Could you check a few things on this drawing? It's one solid part, dimensions in mm from its lowest x, y, z. A direction names the side the tool comes from. Round coordinates to 2 decimals unless told otherwise and drop trailing zeros. Write each loop counter-clockwise with the first axis right and the second up, starting at its lowest first coordinate (ties: lowest second). Pieces come first, ordered by that corner, then holes. Notation, with made-up numbers: (56, 8) -> (70, 8) arc R21 ccw to (70, 36) -> close; hole circle Ø9 at (39.25, -22.5). An arc over 180 degrees is marked (long way). Answer in a Markdown table with one row per item. Add a question column.
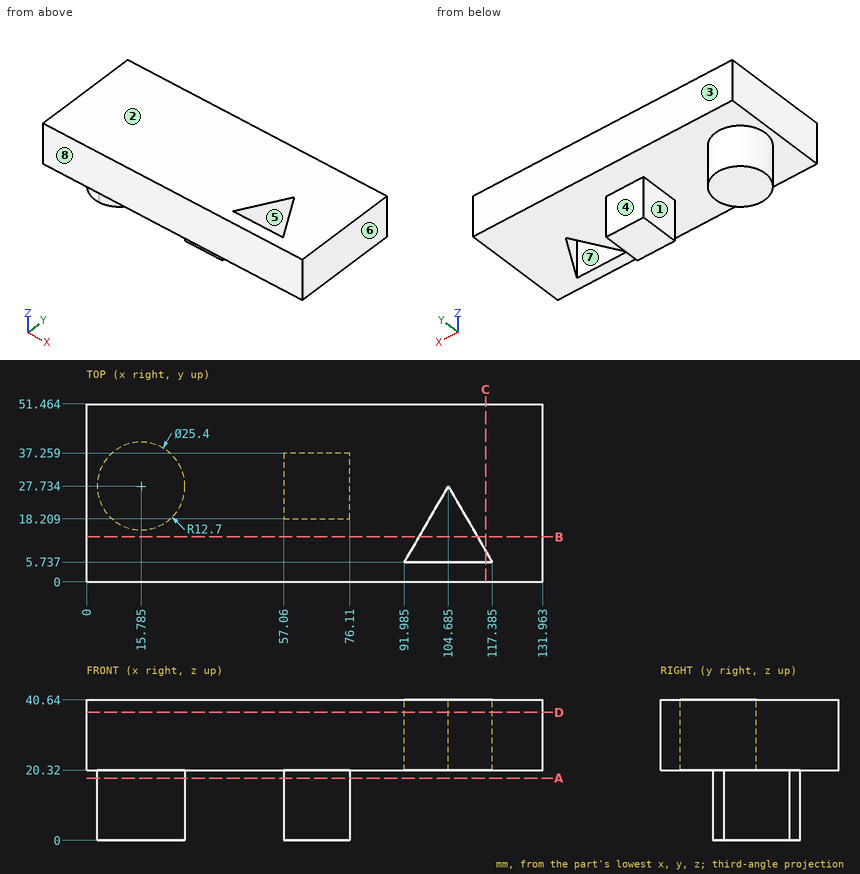
(1) I need wall thicknesses on L1, parallel to Z at x = 80.5, y = 32.5; L2, parallel to X at y = 24.5, z = 26.5; L3, parallel to X at y = 21, z = 3. Which ranges of each line are inside material? Lowest first, please.
(2) Suppose I cut it at D-D, the plane z = 37. Please give me the cut outline in (x, y) (1 decimal).
(3) For P1, Ø5, axis at y = 26.5, z = 17, coming from the -X side (1 decimal); P2, Ø15, axis at y = 25.5, z = 8, coming from the +X side; P3, Ø5.5, axis at x = 66.5, z = 7.5, coming from the -Y side, each with a flat end and sliding along its axis, tell me the tip position at first contact or that it passes through.
(4) If we mould it in two halves opening along Y, with no side actions, what happens to the marked faces 6, 7 and 8? For each: pulls with the +Y half, pulls with the -Y half, needs draft (parallel to the pull), parting line crosses it, or undercut.
(5) On a 3-axis mill with a long thin cutter (end or side, diameter ignored), from which of +Z, -Z, +X, -X, +Y, -Y can I reach the whole of each face in a straight line? I mean the marked faces 1, 2, 3, 4 and 5. Say none if no direction works.
(6) Suppose I cut it at B-B, the plane y = 13. Please give me the cut outline in (x, z), then the cut area to 3 significant figures.
(7) Suppose I cut it at A-A, the plane z = 18. Please give me the cut outline in (x, y) (1 decimal).
(8) Suppose I cut it at C-C, the plane x = 115.5. Please give me the cut outline in (y, z).
Response:
| question | item | result |
|---|---|---|
| 1 | L1 | 20.32 to 40.64 |
| 1 | L2 | 0 to 102.82, 106.55 to 131.96 |
| 1 | L3 | 5.02 to 26.55, 57.06 to 76.11 |
| 2 | outline | (0, 0) -> (132, 0) -> (132, 51.5) -> (0, 51.5) -> close; hole (92, 5.7) -> (117.4, 5.7) -> (104.7, 27.7) -> close |
| 3 | P1 | x = 3.1 |
| 3 | P2 | x = 76.11 |
| 3 | P3 | y = 18.21 |
| 4 | face 6 | needs draft |
| 4 | face 7 | undercut |
| 4 | face 8 | pulls with the -Y half |
| 5 | face 1 | -Z, +Y, -Y |
| 5 | face 2 | +Z, +X, -X, +Y, -Y |
| 5 | face 3 | +Z, -Z, +X, -X, +Y |
| 5 | face 4 | -Z, +X, +Y |
| 5 | face 5 | +Z, -Z |
| 6 | outline | (0, 20.32) -> (96.18, 20.32) -> (96.18, 40.64) -> (0, 40.64) -> close; (113.19, 20.32) -> (131.96, 20.32) -> (131.96, 40.64) -> (113.19, 40.64) -> close |
| 6 | area | 2,340 mm² |
| 7 | outline | circle Ø25.4 at (15.8, 27.7); (57.1, 18.2) -> (76.1, 18.2) -> (76.1, 37.3) -> (57.1, 37.3) -> close |
| 8 | outline | (0, 20.32) -> (5.74, 20.32) -> (5.74, 40.64) -> (0, 40.64) -> close; (9, 20.32) -> (51.46, 20.32) -> (51.46, 40.64) -> (9, 40.64) -> close |
